from build123d import *

# Parameters (mm, degrees)
SKETCH1_W                    = 33.1
SKETCH1_H                    = 27.85
BOSS_EXTRUDE1_DEPTH          = 9.52
SKETCH2_W                    = 13
SKETCH2_H                    = 22.849999999
CUT_EXTRUDE1_DEPTH           = 38.725494033
SKETCH3_W                    = 16
SKETCH3_H                    = 9.5
CUT_EXTRUDE2_DEPTH           = 38.725494033
F_97_0_0059_DIAMETER_HOLE1_D = 2.794


with BuildPart() as part:
    # Sketch1 → Boss-Extrude1 (new body)
    with BuildSketch(Plane.XZ.offset(4.76)):
        with Locations((-7.05, 13.925)):
            Rectangle(SKETCH1_W, SKETCH1_H)
    extrude(amount=-BOSS_EXTRUDE1_DEPTH)

    # Sketch2 → Cut-Extrude1 (cut, through all)
    with BuildSketch(Plane(origin=(0, 4.76, 0), x_dir=(-1, 0, 0), z_dir=(0, 1, 0))):
        with Locations((-3, 16.425)):
            Rectangle(SKETCH2_W, SKETCH2_H)
    extrude(amount=-CUT_EXTRUDE1_DEPTH, mode=Mode.SUBTRACT)

    # Sketch3 → Cut-Extrude2 (cut, through all)
    with BuildSketch(Plane(origin=(0, 4.76, 0), x_dir=(-1, 0, 0), z_dir=(0, 1, 0))):
        with Locations((11.5, 23.1)):
            Rectangle(SKETCH3_W, SKETCH3_H)
    extrude(amount=-CUT_EXTRUDE2_DEPTH, mode=Mode.SUBTRACT)

    # Sketch4 → Cut-Revolve1 (revolve, cut)
    with BuildSketch(Plane(origin=(0, 0, 0), x_dir=(1, 0, 0), z_dir=(0, 1, 0))):
        Polygon((7.2835, 0), (6.5, 0), (6.5, -5.000000001), (7.2835, -5.000000001), (7.2835, -2), align=None)
    revolve(axis=Axis((6.5, 0, 0), (0, 0, 1)), mode=Mode.SUBTRACT)

    # Sketch5 → Cut-Revolve2 (revolve, cut)
    with BuildSketch(Plane(origin=(0, 0, 0), x_dir=(1, 0, 0), z_dir=(0, 1, 0))):
        Polygon((2.2835, 0), (1.5, 0), (1.5, -5.000000001), (2.2835, -5.000000001), (2.2835, -2), align=None)
    revolve(axis=Axis((1.5, 0, 0), (0, 0, 1)), mode=Mode.SUBTRACT)

    # Sketch6 → Cut-Revolve3 (revolve, cut)
    with BuildSketch(Plane.XZ, mode=Mode.PRIVATE) as cut_revolve3_sk:
        Polygon((-13.2705, 18.35), (-14.5, 18.35), (-14.5, 8.35), (-13.2705, 8.35), (-13.2705, 16.35), align=None)
    revolve(cut_revolve3_sk.sketch.rotate(Axis((-14.5, 0, 18.35), (0, 0, -1)), 180), axis=Axis((-14.5, 0, 18.35), (0, 0, -1)), mode=Mode.SUBTRACT)

    # Sketch7 → Cut-Revolve4 (revolve, cut)
    with BuildSketch(Plane.XY.offset(21)):
        Polygon((-23.6, 1.3105), (-23.6, 0), (-19.5, 0), (-19.5, 1.3105), (-21.6, 1.3105), align=None)
    revolve(axis=Axis((-23.6, 0, 21), (1, 0, 0)), mode=Mode.SUBTRACT)

    # #97 (0.0059) Diameter Hole1 (through all)
    with Locations(Plane.ZY.offset(23.6)):
        with Locations((10.71372, 0)):
            Hole(F_97_0_0059_DIAMETER_HOLE1_D / 2)


solid = part.part
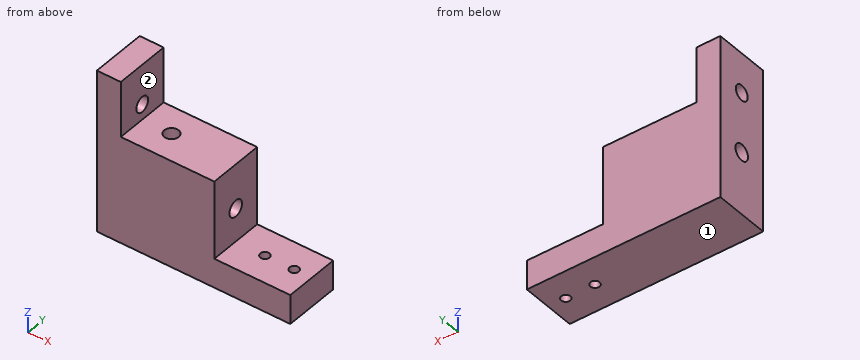
The listing builds one solid part. Answer for the finished solid, in the listing's coordinates (mm). Face numbers are marked on the shaded views. A direction names the side the tool comes from. Coordinates: 2 decimals unless noted, no trailing zeros. Write each loop counter-clockwise with the first axis right and the second up, starting at its lowest first coordinate (ties: lowest second). Pieces come first, ordered by that corner, then holes. Notation, with made-up numbers: (-25, 88) - (-11, 88) arc R24 ccw to (-11, 100) - close; hole circle Ø11 at (70, -18). An arc over 180 degrees is marked (long way). Return JSON: item names as keys, results as strings.
1. The part is cut by section D-D on y = -2.25. Determine the outline of the cut face in (x, z), then the cut area to 3 significant figures.
Final values:
{"outline": "(-23.6, 0) - (9.5, 0) - (9.5, 5) - (-3.5, 5) - (-3.5, 18.35) - (-19.5, 18.35) - (-19.5, 27.85) - (-23.6, 27.85) - close", "area": "473 mm^2"}
2. Each of these flat-tipped pins is pushed along its axis until it touches: pin 1 Ø1.5 at (x, y) = (-14.5, 0) entering from +Z; pin 2 Ø2 at (x, y) = (-17, 0) entering from +Z; pin 3 Ø5 at (x, y) = (1.5, 1.5) entering from +Z. Where does it stop, or does it pass through?
Final values:
{"pin 1": "z = 8.35", "pin 2": "z = 18.35", "pin 3": "z = 5"}
3. The part is cut by section C-C on y = 0. Count the separate pieces of the cut face and the enclosed holes in it, then the cut area to 3 significant figures.
Final values:
{"separate pieces": "6", "enclosed holes": "0", "area": "372 mm^2"}
4. The part is cut by section A-A on z = 21. Determine the outline of the cut face in (x, y).
Final values:
{"outline": "(-23.6, -4.76) - (-19.5, -4.76) - (-19.5, -1.31) - (-23.6, -1.31) - close; (-23.6, 1.31) - (-19.5, 1.31) - (-19.5, 4.76) - (-23.6, 4.76) - close"}
5. The part is cut by section B-B on x = 1.5. Determine the outline of the cut face in (y, z).
Final values:
{"outline": "(-4.76, 0) - (-0.78, 0) - (-0.78, 5) - (-4.76, 5) - close; (0.78, 0) - (4.76, 0) - (4.76, 5) - (0.78, 5) - close"}
6. Consider line 1 along Y through (x, z) = (1.5, 3.8); line 2 along X through (y, z) = (0, 16.75); line 3 along Z through (x, y) = (-7.75, 0). Determine where each line is inside the solid, lowest interval first.
Final values:
{"line 1": "-4.76 to -0.78, 0.78 to 4.76", "line 2": "-23.6 to -15.73, -13.27 to -3.5", "line 3": "0 to 9.32, 12.11 to 18.35"}
7. Which of the six approach directions +Z, -Z, +X, -X, +Y, -Y give full straight-line access (tool end or side, diameter ignored) to the marked faces 1 and 2?
Final values:
{"face 1": "-Z, +X, -X, +Y, -Y", "face 2": "+Z, +X, +Y, -Y"}
